CAD build for the part. Positions are in the model's coordinates, mm. Face numbers are marked on the shaded views. A direction names the side the tool comes from. Give positions to 0.01 mm unless a question says otherwise; leave off trailing zeros. Loops run counter-clockwise (first coordinate to the right, second up) from the corner with the lowest first, then second, coordinate; pieces in that order, holes last. Notation, with made-up numbers: (13, -40) -> (38, -40) arc R28 ccw to (38, -9) -> close; hole circle Ø10 at (-1, -34.75). An arc over 180 degrees is marked (long way). Use one line per item in the form item = value.
```python
from build123d import *

# Parameters (mm, degrees)
BOSS_EXTRUDE1_DEPTH      = 15
SKETCH5_R                = 3
BOSS_EXTRUDE3_DEPTH      = 9.1
SKETCH6_R                = 6
CUT_EXTRUDE1_DEPTH       = 4.2
BOSS_EXTRUDE4_DEPTH      = 1.5
BOSS_EXTRUDE4_DEPTH_BACK = 1.5
SKETCH7_R                = 1


with BuildPart() as part:
    # Sketch1 → Boss-Extrude1 (new body)
    with BuildSketch(Plane.XY):
        Polygon((-2.4, -1.1), (-2.4, 1.1), (-4.4, 1.1), (-4.4, 3.1), (4.4, 3.1), (4.4, 1.1), (2.4, 1.1), (2.4, -1.1), (4.4, -1.1), (4.4, -3.1), (-4.4, -3.1), (-4.4, -1.1), align=None)
    extrude(amount=BOSS_EXTRUDE1_DEPTH)

    # Sketch5 → Boss-Extrude3 (add)
    with BuildSketch(Plane(origin=(0, -1.1, 0), x_dir=(1, 0, 0), z_dir=(0, 1, 0))):
        with BuildLine():
            Line((5.5, -18), (5.5, -12))
            ThreePointArc((5.5, -12), (0, -6.5), (-5.5, -12))
            Line((-5.5, -12), (-5.5, -18))
            ThreePointArc((-5.5, -18), (0, -23.5), (5.5, -18))
        make_face()
        with Locations(Location((0, -18, 0), (0, 0, 180))):
            Circle(SKETCH5_R, mode=Mode.SUBTRACT)
    extrude(amount=-BOSS_EXTRUDE3_DEPTH)

    # Sketch6 → Cut-Extrude1 (cut)
    with BuildSketch(Plane(origin=(0, -8.1, 0), x_dir=(-1, 0, 0), z_dir=(0, -1, 0))):
        with Locations((0, -18)):
            Circle(SKETCH6_R)
    extrude(amount=-CUT_EXTRUDE1_DEPTH, mode=Mode.SUBTRACT)

    # Sketch7 → Boss-Extrude4 (add, two sides: drawn at the far end of the back side and taken through both)
    with BuildSketch(Plane(origin=(0, 0, 0), x_dir=(0, 0, -1), z_dir=(1, 0, 0)).offset(-BOSS_EXTRUDE4_DEPTH_BACK)):
        with BuildLine():
            Line((-3.5, -9.1), (-6.5, -9.1))
            Line((-6.5, -9.1), (-9.5, -9.1))
            Line((-9.5, -9.1), (-9.5, -3.1))
            Line((-9.5, -3.1), (-1, -3.1))
            Line((-1, -3.1), (-1, -6.6))
            ThreePointArc((-1, -6.6), (-1.732233047, -8.367766953), (-3.5, -9.1))
        make_face()
        with Locations((-3.5, -6.6)):
            Circle(SKETCH7_R, mode=Mode.SUBTRACT)
    extrude(amount=BOSS_EXTRUDE4_DEPTH + BOSS_EXTRUDE4_DEPTH_BACK)


solid = part.part
```
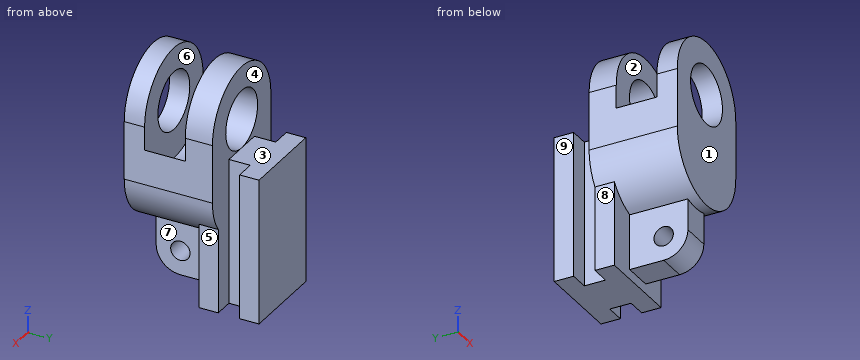
1. Cut at D-D, the plane x = 0.5. Write the cut outline in (y, z).
Result sheet:
outline = (-10.2, 6.52) -> (-9.1, 6.52) -> (-9.1, 3.5) arc R2.5 ccw to (-6.6, 1) -> (-3.1, 1) -> (-3.1, 0) -> (3.1, 0) -> (3.1, 15) -> (-1.1, 15) -> (-1.1, 15.04) -> (-3.9, 15.04) -> (-3.9, 12.02) -> (-8.1, 12.02) -> (-8.1, 15.04) -> (-10.2, 15.04) -> close; (-10.2, 20.96) -> (-8.1, 20.96) -> (-8.1, 23.48) -> (-10.2, 23.48) -> close; (-3.9, 20.96) -> (-1.1, 20.96) -> (-1.1, 23.48) -> (-3.9, 23.48) -> close; hole circle Ø2 at (-6.6, 3.5)
2. Cut at A-A, the plane y = -2. Write the cut outline in (x, z).
Result sheet:
outline = (-5.5, 12) arc R5.5 ccw to (-4.4, 8.7) -> (-4.4, 0) -> (4.4, 0) -> (4.4, 8.7) arc R5.5 ccw to (5.5, 12) -> (5.5, 18) arc R5.5 ccw to (-5.5, 18) -> close; hole circle Ø6 at (0, 18)
3. Drop flat-ended pins along their axis: P1, Ø2.5, axis at y = -6.6, z = 3.5, coming from the +X side; P2, Ø1.5, axis at x = -1, y = -8, coming from the +Z side; P3, Ø2.5, axis at y = -0.5, z = 7, coming from the -X side. Give the stop position or say it passes through.
Result sheet:
P1 = 1.5
P2 = 23.49
P3 = -4.4
4. Mould opens along Y. For the marked faces 1, 2, 3 and 4 say: pulls with the +Y half, pulls with the -Y half, needs draft (parallel to the pull), parting line crosses it, or undercut.
Result sheet:
face_1 = pulls with the -Y half
face_2 = undercut
face_3 = needs draft
face_4 = undercut
5. Drill centre lines: line 1 (Y direction, x = -3.5, z = 13.5); line 2 (Y direction, x = 2.5, z = 6.5); line 3 (Y direction, x = 0.5, z = 14.5). Where is each one in solid material? Low to high.
Result sheet:
line_1 = -10.2 to -8.1, -3.9 to -1.1, 1.1 to 3.1
line_2 = -3.1 to -1.1, 1.1 to 3.1
line_3 = -10.2 to -8.1, -3.9 to 3.1
6. Cut at B-B, the plane z = 14. Write the cut outline in (x, y).
Result sheet:
outline = (-5.5, -10.2) -> (5.5, -10.2) -> (5.5, -1.1) -> (2.4, -1.1) -> (2.4, 1.1) -> (4.4, 1.1) -> (4.4, 3.1) -> (-4.4, 3.1) -> (-4.4, 1.1) -> (-2.4, 1.1) -> (-2.4, -1.1) -> (-5.5, -1.1) -> close; hole (-4.47, -8.1) -> (4.47, -8.1) -> (4.47, -3.9) -> (-4.47, -3.9) -> close
7. Cut at C-C, the plane y = -7.25. Write the cut outline in (x, z).
Result sheet:
outline = (-5.5, 12) arc R5.5 ccw to (-1.5, 6.71) -> (-1.5, 4.26) -> (1.5, 4.26) -> (1.5, 6.71) arc R5.5 ccw to (5.5, 12) -> (5.5, 15.6) arc R6 cw to (-5.5, 15.6) -> close; (-1.5, 1.09) -> (1.5, 1.09) -> (1.5, 2.74) -> (-1.5, 2.74) -> close
8. Tool access for the marked faces 5, 6, 7, 8 and 9: list every direction of +Z, -Z, +X, -X, +Y, -Y with a clear straight run to the whole face (end or side of a thin tool).
Result sheet:
face_5 = -Z, +X, +Y, -Y
face_6 = +Z
face_7 = -Z, +X, -Y
face_8 = -Z, -X, +Y, -Y
face_9 = +Z, -Z, -X, +Y
